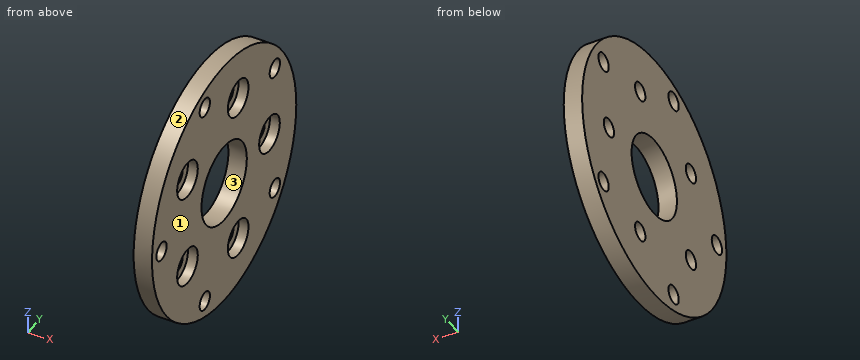
Autodesk Inventor part; units mm, degrees
ref_plane "YZ Plane" through (0, 0, 0) normal (1, 0, 0) x (0, 1, 0)
ref_plane "XZ Plane" through (0, 0, 0) normal (0, 1, 0) x (-1, 0, 0)
ref_plane "XY Plane" through (0, 0, 0) normal (0, 0, 1) x (1, 0, 0)
sketch "Sketch1" plane through (0, 0, 0) normal (1, 0, 0) x (0, 1, 0)
  circle A0 centre (0, 0) radius 13.97
  circle A1 centre (0, 0) radius 44.45
  dimension "d0" = 27.94
  dimension "d1" = 88.9
extrude "Extrusion1" add sketch "Sketch1" along normal blind 6.35
sketch "Sketch2" plane through (6.35, 0, 0) normal (1, 0, 0) x (0, 0, -1)
  arc A0 (25.458, -0.8256) -> (35.4837, 5.2699) centre (26.5725, 8.6339) ccw
  arc A1 (25.6093, -25.1202) -> (21.0812, -14.2959) centre (16.4227, -22.6039) ccw
  arc A2 (37.0087, -36.5562) -> (51.4278, 7.8214) centre (0, 0) ccw
  circle A3 centre (36.7212, -11.9315) radius 13.4082
  circle A4 centre (36.7212, -11.9315) radius 3.175
  circle A5 centre (22.695, 31.237) radius 3.175
  circle A6 centre (-22.695, 31.237) radius 3.175
  circle A7 centre (-36.7212, -11.9315) radius 3.175
  circle A8 centre (0, -38.611) radius 3.175
  point P0 (0, 0)
  dimension "d4" = 6.35
  dimension "d7" = 360
extrude "Extrusion2" cut sketch "Sketch2" against normal through all contours A4 | A5 | A6 | A7 | A8
thread "Thread1"
thread "Thread2"
thread "Thread3"
thread "Thread4"
thread "Thread5"
sketch "Sketch3" plane through (6.35, 0, 0) normal (1, 0, 0) x (0, 0, -1)
  circle A0 centre (26.5725, 8.6339) radius 1.27
  circle A1 centre (26.5725, 8.6339) radius 3.175
  circle A2 centre (0, 27.94) radius 3.175
  circle A3 centre (-26.5725, 8.6339) radius 3.175
  circle A4 centre (-16.4227, -22.6039) radius 3.175
  circle A5 centre (16.4227, -22.6039) radius 3.175
  point P0 (0, 0)
  dimension "d21" = 6.35
  dimension "d24" = 360
extrude "Extrusion3" cut sketch "Sketch3" against normal up to next contours A0 | A1 | A2 | A3 | A4 | A5
sketch "Sketch4" plane through (6.35, 0, 0) normal (1, 0, 0) x (0, 0, -1)
  circle A0 centre (26.5725, 8.6339) radius 3.175
  circle A1 centre (26.5725, 8.6339) radius 6.35
  circle A2 centre (0, 27.94) radius 6.35
  circle A3 centre (-26.5725, 8.6339) radius 6.35
  circle A4 centre (-16.4227, -22.6039) radius 6.35
  circle A5 centre (16.4227, -22.6039) radius 6.35
  point P0 (0, 0)
  dimension "d28" = 12.7
  dimension "d33" = 360
extrude "Extrusion4" cut sketch "Sketch4" against normal blind 3.429
properties part number "spacer_flange"
Geometry check sheet. Reference: the model listing, model coordinates, mm. Face numbers are marked on the shaded views. Give positions to 0.01 mm unless a question says otherwise; leave off trailing zeros. Write each loop counter-clockwise with the first axis right and the second up, starting at its lowest first coordinate (ties: lowest second). Pieces come first, ordered by that corner, then holes. Notation, with made-up numbers: M 70.25,27.25 L 92.25,27.25 A24 cw 92.25,53.25 Z; hole C 7,-12.5 d7. An arc over 180 degrees is marked long. One line per question, with ' | ' between items.
1. Cross-section at B-B (z = 0). Enter the section's corners in (x, y) (3 decimals).
Ans:
outline: M 0,-44.45 L 6.35,-44.45 L 6.35,-41.786 L 0,-41.786 Z; M 0,-35.436 L 6.35,-35.436 L 6.35,-13.97 L 0,-13.97 Z; M 0,13.97 L 6.35,13.97 L 6.35,21.59 L 2.921,21.59 L 2.921,24.765 L 0,24.765 Z; M 0,31.115 L 2.921,31.115 L 2.921,34.29 L 6.35,34.29 L 6.35,44.45 L 0,44.45 Z
2. Scan lines: line 1 along Z through (x, y) = (4, -24); line 2 along Z through (x, y) = (4.75, -19); line 3 along Y through (x, z) = (1.5, -20). Record each from-to range of solid material in increasing order. Write a range as from..to.
Ans:
line 1: -37.41..-22.62, -10.23..10.23, 22.62..37.41 | line 2: -40.18..-21.65, -11.19..11.19, 21.65..40.18 | line 3: -39.7..29.56, 32.92..39.7
3. Mould release check, pull along Z, two halves, no side actions. Record for the marked faces 1, 2 and 3: released by +Z, released by -Z, zero draft, split by the parting line, or undercut.
Ans:
face 1: zero draft | face 2: split by the parting line | face 3: undercut
4. Gauge pin test, flat ends, axial feed: pin 1 (4 mm diameter, centred on y = 6, z = 29.5, fed in from +X); pin 2 (4 mm diameter, centred on y = 31.237, z = -22.695, fed in from +X); pin 3 (1 mm diameter, centred on x = 0.5, y = -25, fed in from +Z); pin 4 (3 mm diameter, centred on x = 3, z = 5, fed in from -Y). Record the tip position at first contact, or that the pin passes through.
Ans:
pin 1: x = 2.92 | pin 2: through | pin 3: z = 37.09 | pin 4: y = -44.31
5. Cross-section at A-A (y = 0). Enter the section's corners in (x, z).
Ans:
outline: M 0,-44.45 L 6.35,-44.45 L 6.35,-13.97 L 0,-13.97 Z; M 0,13.97 L 6.35,13.97 L 6.35,44.45 L 0,44.45 Z
6. Cross-section at C-C (y = 37.5). Enter the section's corners in (x, z), plus the area to 3 significant figures.
Ans:
outline: M 0,-23.87 L 6.35,-23.87 L 6.35,23.87 L 0,23.87 Z | area: 303 mm2
